Build history of the part. All positions in model axes, mm. A direction names the side the tool comes from. Give positions to 0.01 mm unless a question says otherwise; leave off trailing zeros. Order: outer loops, then holes, each group sorted by start corner. A loop starts at its lowest first (then second) coordinate and runs counter-clockwise, first axis right, second up. Notation, with made-up numbers: (72.25, 52) -> (88.25, 52) arc R5 ccw to (88.25, 61) -> close; hole circle Ø3 at (46, 13.5). An arc over 180 degrees is marked (long way). One line per item, written item: value. Start each with the question number.
(1) Saw through at C-C on z = -2.6. Give the cut face in (x, y).
(2) Which spindle directions (+Z, -Z, +X, -X, +Y, -Y) get a long thin tool onto all of the face, cutting with end or side? Do faces 1 (the flat face through (-3, -3, -0.4)), 2 (the cylindrical face through (4.38, -8.43, 0.76)). Say none if no direction does.
(3) Pin check, flat tips, straight feed: pin 1 (6.5 mm diameter, centred on x = -1, y = 0.5, fed in from +Z); pin 2 (3.5 mm diameter, centred on x = -2.5, y = -2, fed in from -Z). Stop position of each tip, or through.
(4) Saw through at A-A on y = 0. Give the cut face in (x, z).
(5) Probe line 1 (Z direction, x = 2, y = 8.5); line 2 (Z direction, x = 2.25, y = -1.25); line 3 (X direction, y = -6.25, z = 0.7). List the from-to ranges inside material, lowest first.
(6) Two-plate mould, pull along Y, no slides. Class faces 3 (the flat face through (0, 0, 1.8)), 4 (the cylindrical face through (-3.047, 0.134, -1.632)), 5 (the flat face through (0, 0, -2.9)): +Y half, -Y half, draft (parallel to the pull), parting line (faces both ways), or undercut.
```python
from build123d import *

# Parameters (mm, degrees)
F0_W   = 3.05
F0_H   = 0.4
F0_W_2 = 2.95
F0_H_2 = 2.5
F2_R   = 0.5


# Not quite as in the source:
# - a fillet or chamfer that OpenCascade refuses, or shapes differently, is made with other operations: its cross-section is extruded or revolved along the edge and cut away or added
# - a feature names something its author has since deleted; it is built from what else it names


with BuildPart() as f1:
    # F0 (on Front) → F1 (revolve)
    with BuildSketch(Plane.XZ):
        Polygon((0, 1.8), (0, 0), (3.05, 0), (6, 0), (9.5, 0), (9.5, 2), (4, 2), (4, 1.8), align=None)
        with Locations((1.525, -0.2)):
            Rectangle(F0_W, F0_H)
        with Locations((4.525, -0.2)):
            Rectangle(F0_W_2, F0_H)
        with Locations((1.525, -1.65)):
            Rectangle(F0_W, F0_H_2)
    revolve(axis=Axis((0, 0, 0.9), (0, 0, 1)))

    # F2
    f2_edges = [f1.edges().sort_by_distance(p)[0] for p in [
        (-9.5, 0, 2),
    ]]
    fillet(f2_edges, radius=F2_R)

    # F3: fillet of radius 1 on 1 edges, made by hand

    # F3_s1 → F3_t2 (revolve, cut)
    with BuildSketch(Plane.XZ):
        with BuildLine():
            ThreePointArc((4.6, 2), (4.283772234, 1.9486832981), (4, 1.8))
            Line((4, 1.8), (4, 2))
            Line((4, 2), (4.6, 2))
        make_face()
    revolve(axis=Axis((0, 0, 2), (0, 0, 1)), mode=Mode.SUBTRACT)


solid = f1.part
```
Results below:
1. outline: circle Ø6.1 at (0, 0)
2. face 1: -Z
2. face 2: +Z, -Z
3. pin 1: stops at z = 1.97
3. pin 2: stops at z = -2.9
4. outline: (-9.5, 0) -> (-6, 0) -> (-6, -0.4) -> (-3.05, -0.4) -> (-3.05, -2.9) -> (3.05, -2.9) -> (3.05, -0.4) -> (6, -0.4) -> (6, 0) -> (9.5, 0) -> (9.5, 1.5) arc R0.5 ccw to (9, 2) -> (4.6, 2) arc R1 ccw to (4, 1.8) -> (-4, 1.8) arc R1 ccw to (-4.6, 2) -> (-9, 2) arc R0.5 ccw to (-9.5, 1.5) -> close
5. line 1: z = 0 to 2
5. line 2: z = -2.9 to 1.8
5. line 3: x = -7.15 to 7.15
6. face 3: undercut
6. face 4: parting line
6. face 5: draft
